```python
from build123d import *

# Parameters (mm, degrees)
F0_W     = 609.6
F0_H     = 609.6
F0_W_2   = 76.2
F0_H_2   = 76.2
F0_W_3   = 406.4
F0_H_3   = 406.4
F1_DEPTH = 38.1
F2_DEPTH = 76.2
F3_DEPTH = 762
F6_DEPTH = 38.1


with BuildPart() as f1:
    # F0 (on Top) → F1 (new body)
    with BuildSketch(Plane.XY):
        Rectangle(F0_W, F0_H)
        Polygon((203.2, 279.4), (279.4, 279.4), (279.4, 203.2), (279.4, -203.2), (279.4, -279.4), (203.2, -279.4), (-203.2, -279.4), (-279.4, -279.4), (-279.4, -203.2), (-279.4, 203.2), (-279.4, 279.4), (-203.2, 279.4), align=None, mode=Mode.SUBTRACT)
        with Locations((-241.3, 241.3)):
            Rectangle(F0_W_2, F0_H_2)
        with Locations((0, 241.3)):
            Rectangle(F0_W_3, F0_H_2)
        with Locations((241.3, 241.3)):
            Rectangle(F0_W_2, F0_H_2)
        with Locations((241.3, 0)):
            Rectangle(F0_W_2, F0_H_3)
        with Locations((241.3, -241.3)):
            Rectangle(F0_W_2, F0_H_2)
        with Locations((0, -241.3)):
            Rectangle(F0_W_3, F0_H_2)
        with Locations((-241.3, -241.3)):
            Rectangle(F0_W_2, F0_H_2)
        with Locations((-241.3, 0)):
            Rectangle(F0_W_2, F0_H_3)
        Rectangle(F0_W_3, F0_H_3)
    extrude(amount=-F1_DEPTH)

    # F0 (on Top) → F2 (join)
    with BuildSketch(Plane.XY):
        with Locations((-241.3, -241.3)):
            Rectangle(F0_W_2, F0_H_2)
        with Locations((-241.3, 0)):
            Rectangle(F0_W_2, F0_H_3)
        with Locations((0, -241.3)):
            Rectangle(F0_W_3, F0_H_2)
        with Locations((241.3, -241.3)):
            Rectangle(F0_W_2, F0_H_2)
        with Locations((241.3, 0)):
            Rectangle(F0_W_2, F0_H_3)
        with Locations((241.3, 241.3)):
            Rectangle(F0_W_2, F0_H_2)
        with Locations((0, 241.3)):
            Rectangle(F0_W_3, F0_H_2)
        with Locations((-241.3, 241.3)):
            Rectangle(F0_W_2, F0_H_2)
    extrude(amount=-F2_DEPTH)

    # F0 (on Top) → F3 (join)
    with BuildSketch(Plane.XY):
        with Locations((-241.3, 241.3)):
            Rectangle(F0_W_2, F0_H_2)
        with Locations((-241.3, -241.3)):
            Rectangle(F0_W_2, F0_H_2)
        with Locations((241.3, -241.3)):
            Rectangle(F0_W_2, F0_H_2)
        with Locations((241.3, 241.3)):
            Rectangle(F0_W_2, F0_H_2)
    extrude(amount=-F3_DEPTH)

    # F5 (on face) → F6 (join)
    with BuildSketch(Plane.XY):
        with BuildLine():
            ThreePointArc((-304.8, 304.8), (-609.6, 0), (-304.8, -304.8))
            Line((-304.8, -304.8), (-304.8, 304.8))
        make_face()
    extrude(amount=-F6_DEPTH)


solid = f1.part
```
Work out the finished part from the listing and answer in its coordinate system (mm). A direction names the side the tool comes from. Round coordinates to 2 decimals unless told otherwise and drop trailing zeros. Loops run counter-clockwise (first coordinate to the right, second up) from the corner with the lowest first, then second, coordinate; pieces in that order, holes last. Notation, with made-up numbers: M 21.5,33 L 77.5,33 A13 cw 77.5,44 Z; hole C 73.25,-33 d5. An arc over 180 degrees is marked long. Use CSV: the item, a comma, the result in double quotes.
Q1. Section A-A, the plane z = -407 is taken. Determine the outline of the cut face in (x, y).
Determined:
outline,"M -279.4,-279.4 L -203.2,-279.4 L -203.2,-203.2 L -279.4,-203.2 Z; M -279.4,203.2 L -203.2,203.2 L -203.2,279.4 L -279.4,279.4 Z; M 203.2,-279.4 L 279.4,-279.4 L 279.4,-203.2 L 203.2,-203.2 Z; M 203.2,203.2 L 279.4,203.2 L 279.4,279.4 L 203.2,279.4 Z"
Q2. Each of these flat-tipped pins is pushed along its axis until it touches: pin 1 (4 mm diameter, centred on x = 81, y = 92, fed in from -Z); pin 2 (11.5 mm diameter, centred on y = -37, z = -64, fed in from -X). Where does it stop, or does it pass through?
Determined:
pin 1,"z = -38.1"
pin 2,"x = -279.4"
Q3. Consider L1, parallel to X at y = 169.5, z = -41; L2, parallel to Z at x = -128, y = 3. Determine where each line is inside the solid, lowest interval first.
Determined:
L1,"-279.4 to -203.2, 203.2 to 279.4"
L2,"-38.1 to 0"
Q4. Section B-B, the plane x = -230 is taken. Determine the outline of the cut face in (y, z).
Determined:
outline,"M -304.8,-38.1 L -279.4,-38.1 L -279.4,-762 L -203.2,-762 L -203.2,-76.2 L 203.2,-76.2 L 203.2,-762 L 279.4,-762 L 279.4,-38.1 L 304.8,-38.1 L 304.8,0 L -304.8,0 Z"
Q5. Section C-C, the plane y = 0 is taken. Determine the outline of the cut face in (x, z), then the cut area to 3 significant figures.
Determined:
outline,"M -609.6,-38.1 L -279.4,-38.1 L -279.4,-76.2 L -203.2,-76.2 L -203.2,-38.1 L 203.2,-38.1 L 203.2,-76.2 L 279.4,-76.2 L 279.4,-38.1 L 304.8,-38.1 L 304.8,0 L -609.6,0 Z"
area,"40,600 mm2"
Q6. The mould has two halves that part along Y. Classify faces 1 (the flat face through (-208, -279.4, -398)), 2 (the flat face through (-159, 4, 0)), 3 (the flat face through (-242, 203.2, -414)): pulls with the +Y half, pulls with the -Y half, needs draft (parallel to the pull), parting line crosses it, or undercut.
Determined:
face 1,"pulls with the -Y half"
face 2,"needs draft"
face 3,"undercut"
Q7. A tool of negligible diameter and unlimited length cuts with its end or side. For faces 4 (the flat face through (241, -203.2, -414)), 5 (the flat face through (-203.2, 241, -414)), 6 (the flat face through (-203.2, -3, -57)), from which of +Z, -Z, +X, -X, +Y, -Y can it reach the whole face along a straight path? Write none if from no direction.
Determined:
face 4,"-Z, +X, -X"
face 5,"-Z, +Y, -Y"
face 6,"-Z"
